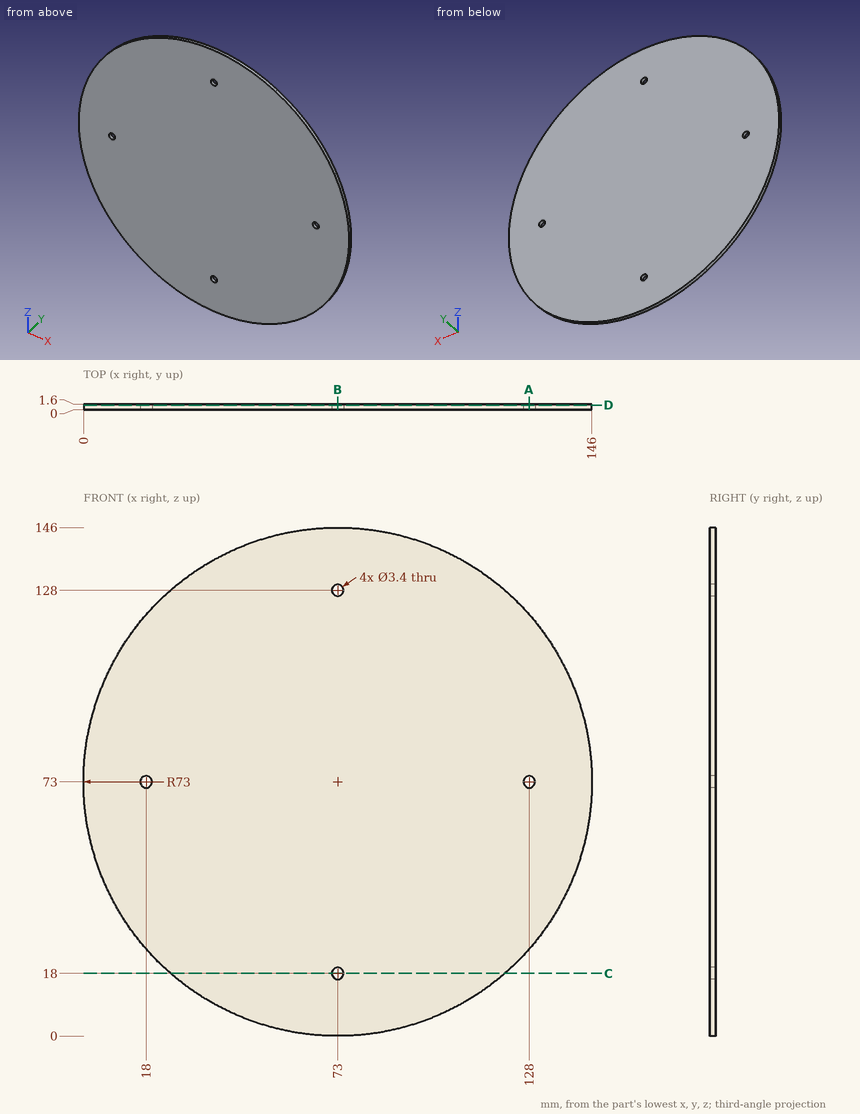
Geometry check sheet. Reference: drawing and pictorial views, mm from the part's lowest x, y, z. Give positions to 0.01 mm unless a question says otherwise; leave off trailing zeros. Write each loop counter-clockwise with the first axis right and the second up, starting at its lowest first coordinate (ties: lowest second). Pieces come first, ordered by that corner, then holes.
Item 1: Cross-section at A-A (x = 128). Enter the section's corners in (y, z).
Item 2: Cross-section at B-B (x = 73). Enter the section's corners in (y, z).
Item 3: Scan lines: L1, parallel to X at y = 0.8, z = 73; L2, parallel to Z at x = 128, y = 0.7. Record each from-to range of solid material in increasing order.
Item 4: Cross-section at C-C (z = 18). Enter the section's corners in (x, y), and give its area (3 significant figures).
Item 5: Cross-section at D-D (y = 1.3). Enter the section's corners in (x, z), and give its area (3 significant figures).
Report:
1. outline: (0, 25) - (1.6, 25) - (1.6, 71.3) - (0, 71.3) - close; (0, 74.7) - (1.6, 74.7) - (1.6, 121) - (0, 121) - close
2. outline: (0, 0) - (1.6, 0) - (1.6, 16.3) - (0, 16.3) - close; (0, 19.7) - (1.6, 19.7) - (1.6, 126.3) - (0, 126.3) - close; (0, 129.7) - (1.6, 129.7) - (1.6, 146) - (0, 146) - close
3. L1: x = 0 to 16.3, 19.7 to 126.3, 129.7 to 146
3. L2: z = 25 to 71.3, 74.7 to 121
4. outline: (25, 0) - (71.3, 0) - (71.3, 1.6) - (25, 1.6) - close; (74.7, 0) - (121, 0) - (121, 1.6) - (74.7, 1.6) - close
4. area: 148 mm2
5. outline: circle Ø146 at (73, 73); hole circle Ø3.4 at (18, 73); hole circle Ø3.4 at (73, 18); hole circle Ø3.4 at (73, 128); hole circle Ø3.4 at (128, 73)
5. area: 16,700 mm2
